Job drawing, mm, ordinate dimensions from the low corner. One solid piece. A direction names the side the tool comes from. Give positions to 0.01 mm unless a question says otherwise; leave off trailing zeros. Loops run counter-clockwise (first coordinate to the right, second up) from the corner with the lowest first, then second, coordinate; pieces in that order, holes last. Notation, with made-up numbers: (7.25, 11.5) - (29.25, 11.5) arc R27 ccw to (29.25, 29.5) - close; hole circle Ø5 at (-31, 71.5). An arc over 180 degrees is marked (long way). Use a Markdown table: item, result.
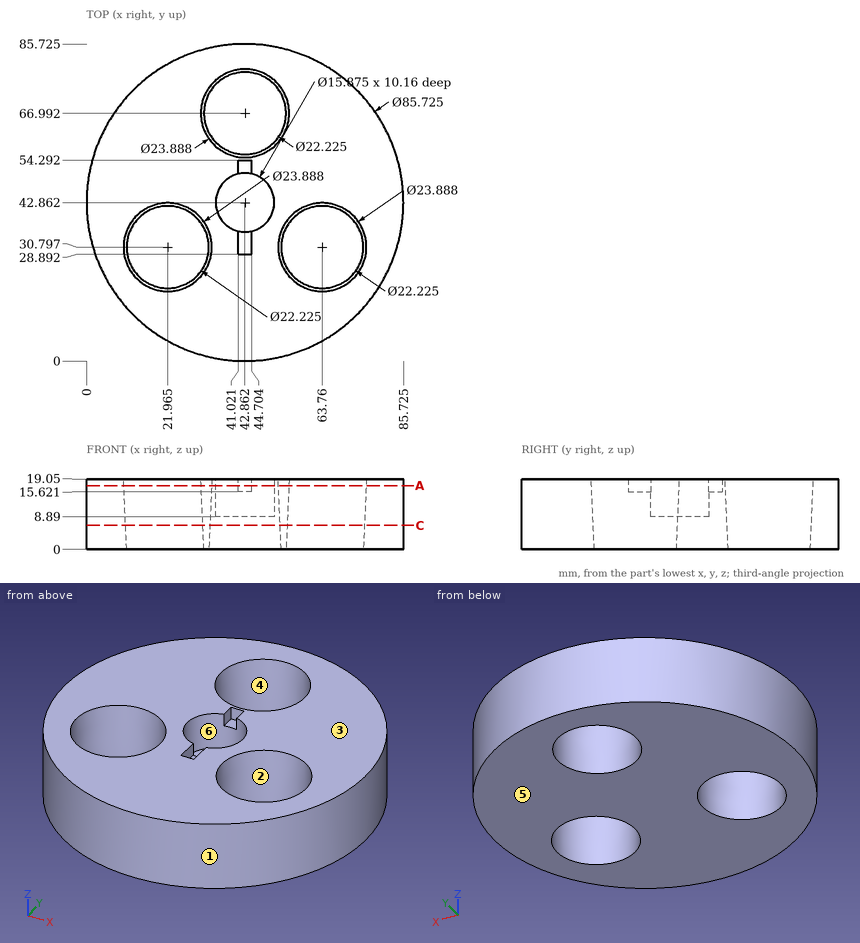
(1) Drill centre lines: probe 1 along Y at (x, z) = (42, 14.5); probe 2 along Z at (x, y) = (49, 45.5); probe 3 along Y at (x, z) = (34.5, 1) (1 decimal). Where is each one in solid material? Low to high. Write a range as [from, to].
Computed:
| item | result |
|---|---|
| probe 1 | [0.01, 34.97], [50.75, 55.28], [78.71, 85.72] |
| probe 2 | [0, 8.89] |
| probe 3 | [0.8, 59.6], [74.4, 84.9] |
(2) 3-axis set-ups, long thin cutter, end or side, ignore diameter. For the marked faces 5 and 6: which of +Z, -Z, +X, -X, +Y, -Y reach the whole face in a straight line?
Computed:
| item | result |
|---|---|
| face 5 | -Z, +X, -X, +Y, -Y |
| face 6 | +Z |
(3) Mould opens along Y. For the marked faces 1, 2, 3 and 4 say: pulls with the +Y half, pulls with the -Y half, needs draft (parallel to the pull), parting line crosses it, or undercut.
Computed:
| item | result |
|---|---|
| face 1 | parting line crosses it |
| face 2 | undercut |
| face 3 | needs draft |
| face 4 | undercut |
(4) Slice it at A-A, the plane z = 17.25. Write the cut outline in (x, y) (1 decimal).
Computed:
| item | result |
|---|---|
| outline | circle Ø85.7 at (42.9, 42.9); hole circle Ø23.7 at (22, 30.8); hole circle Ø23.7 at (42.9, 67); hole (41, 28.9) - (44.7, 28.9) - (44.7, 35.1) arc R7.9 ccw to (44.7, 50.6) - (44.7, 54.3) - (41, 54.3) - (41, 50.6) arc R7.9 ccw to (41, 35.1) - close; hole circle Ø23.7 at (63.8, 30.8) |
(5) Slice it at C-C, the plane z = 6.5. Write the cut outline in (x, y) (1 decimal).
Computed:
| item | result |
|---|---|
| outline | circle Ø85.7 at (42.9, 42.9); hole circle Ø22.8 at (22, 30.8); hole circle Ø22.8 at (42.9, 67); hole circle Ø22.8 at (63.8, 30.8) |
(6) Pin check, flat tips, straight feed: P1, Ø1.1, axis at x = 43.5, y = 52.5, coming from the +Z side; P2, Ø4, axis at y = 21.5, z = 5.5, coming from the -X side; P3, Ø4, axis at y = 51.5, z = 17.5, coming from the +X side. Stop position of each tip, or through.
Computed:
| item | result |
|---|---|
| P1 | z = 15.62 |
| P2 | x = 4.62 |
| P3 | x = 85.21 |
